Verification items for the finished model (mm, model axes). Face numbers are marked on the shaded views. A direction names the side the tool comes from. Round coordinates to 2 decimals unless told otherwise and drop trailing zeros. Order: outer loops, then holes, each group sorted by start corner. A loop starts at its lowest first (then second) coordinate and runs counter-clockwise, first axis right, second up. Notation, with made-up numbers: (75, 22.25) -> (108, 22.25) arc R35 cw to (108, 56.25) -> close; hole circle Ø4 at (-28, 4). An arc over 180 degrees is marked (long way). Return JSON: item names as keys, results as strings. Group by question number.
Item 1: Sectioned sample at D-D on z = 2.25. Record the cut outline in (x, y).
Item 2: Scan lines: probe 1 along Y at (x, z) = (0, 6.25); probe 2 along Y at (x, z) = (0, 3); probe 3 along X at (y, z) = (0, 3.75). Record each from-to range of solid material in increasing order. Write a range as from..to.
Item 3: Sectioned sample at B-B on x = -8. Record the cut outline in (y, z), plus the area to 4 significant figures.
Item 4: Depth check by flat-ended pin: pin 1 Ø1.5 at (x, z) = (7.5, -3) entering from +Y; pin 2 Ø1 at (y, z) = (-1, -1) entering from -X; pin 3 Ø3 at (x, z) = (-6, -4.5) entering from -Y. Enter the tip coordinate at first touch or a pass-through.
Item 5: Sectioned sample at A-A on z = 9. Record the cut outline in (x, y), plus the area to 3 significant figures.
Item 6: Access from +Z, -Z, +X, -X, +Y, -Y to the whole of each face (thin tool, end or side, straight path). Record for the marked faces 1, 2 and 3.
Item 7: Sectioned sample at C-C on y = 0. Record the cut outline in (x, z), plus the area to 3 significant figures.
Item 8: Draft check along X on the marked faces 4, 5, 6 and 7. Enter one of: pulls with the +X half, pulls with the -X half, needs draft (parallel to the pull), parting line crosses it, or undercut.
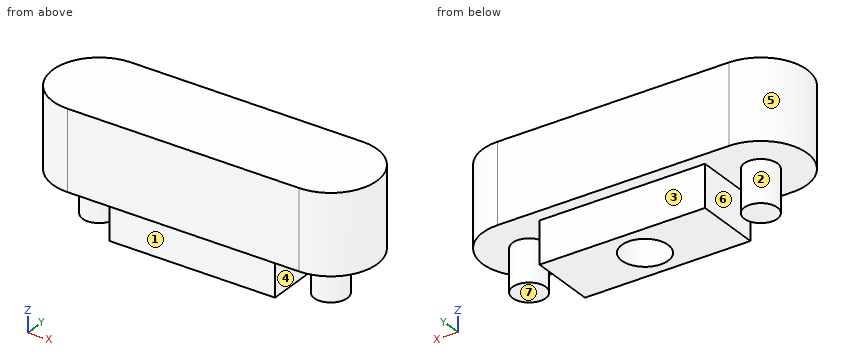
Autodesk Inventor part; units mm, degrees
ref_plane "YZ Plane" through (0, 0, 0) normal (1, 0, 0) x (0, 1, 0)
ref_plane "XZ Plane" through (0, 0, 0) normal (0, 1, 0) x (-1, 0, 0)
ref_plane "XY Plane" through (0, 0, 0) normal (0, 0, 1) x (1, 0, 0)
sketch "Sketch1" plane through (0, 0, 0) normal (0, 0, 1) x (1, 0, 0)
  circle A0 centre (17.5, 0) radius 2.5
  circle A1 centre (-17.5, 0) radius 2.5
  line L0 (17.5, -7) -> (-17.5, -7)
  arc A2 (-17.5, 7) -> (-17.5, -7) centre (-17.5, 0) ccw
  line L1 (-17.5, 7) -> (17.5, 7)
  arc A3 (17.5, -7) -> (17.5, 7) centre (17.5, 0) ccw
  line L2 (-12.5, -5) -> (12.5, -5)
  line L3 (12.5, 5) -> (-12.5, 5)
  circle A4 centre (0, 0) radius 3.5
  dimension "d0" = 2
  dimension "d1" = 17.5
  dimension "d2" = 7
extrude "Extrusion1" add sketch "Sketch1" along normal blind 10 contours A0 | A1 | L0 A2 L1 A3
sketch "Sketch2" plane through (0, 0, 10) normal (0, 0, 1) x (1, 0, 0)
  arc A0 (17.5, -7) -> (17.5, 7) centre (17.5, 0) ccw
  line L0 (-17.5, -7) -> (17.5, -7)
  arc A1 (-17.5, 7) -> (-17.5, -7) centre (-17.5, 0) ccw
  line L1 (17.5, 7) -> (-17.5, 7)
  point P0 (0, 0)
extrude "Extrusion2" add sketch "Sketch2" along normal blind 2
sketch "Sketch3" plane through (0, 0, 10) normal (0, 0, -1) x (-1, 0, 0)
  circle A0 centre (0, 0) radius 1.7
  dimension "d7" = 3.4
extrude "Extrusion3" add sketch "Sketch3" along normal blind 5
sketch "Sketch4" plane through (0, 0, 0) normal (0, 0, -1) x (-1, 0, 0)
  circle A0 centre (17.5, 0) radius 2.5
  line L0 (12.5, 5) -> (12.5, -5)
  line L1 (-12.5, 5) -> (12.5, 5)
  line L2 (12.5, -5) -> (-12.5, -5)
  line L3 (-12.5, -5) -> (-12.5, 5)
  circle A1 centre (0, 0) radius 3.5
  circle A2 centre (-17.5, 0) radius 2.5
extrude "Extrusion4" add sketch "Sketch4" along normal blind 6.35
properties part number "SpringHolderV1"
Recorded:
{
 "1": {"outline": "(-17.5, -7) -> (17.5, -7) arc R7 ccw to (17.5, 7) -> (-17.5, 7) arc R7 ccw to start; hole circle Ø7 at (0, 0)"},
 "2": {"probe 1": "-7..-3.5, -1.7..1.7, 3.5..7", "probe 2": "-7..-3.5, 3.5..7", "probe 3": "-24.5..-3.5, 3.5..24.5"},
 "3": {"outline": "(-7, 0) -> (-5, 0) -> (-5, -6.35) -> (5, -6.35) -> (5, 0) -> (7, 0) -> (7, 12) -> (-7, 12) -> close", "area": "231.5 mm²"},
 "4": {"pin 1": "y = 5", "pin 2": "x = -19.95", "pin 3": "y = -5"},
 "5": {"outline": "(-17.5, -7) -> (17.5, -7) arc R7 ccw to (17.5, 7) -> (-17.5, 7) arc R7 ccw to start; circle Ø3.4 at (0, 0); hole circle Ø7 at (0, 0)", "area": "615 mm²"},
 "6": {"face 1": "-Z, +X, -X, -Y", "face 2": "-Z", "face 3": "-Z, +X, -X, +Y"},
 "7": {"outline": "(-24.5, 0) -> (-20, 0) -> (-20, -6.35) -> (-15, -6.35) -> (-15, 0) -> (-12.5, 0) -> (-12.5, -6.35) -> (-3.5, -6.35) -> (-3.5, 10) -> (-1.7, 10) -> (-1.7, 5) -> (1.7, 5) -> (1.7, 10) -> (3.5, 10) -> (3.5, -6.35) -> (12.5, -6.35) -> (12.5, 0) -> (15, 0) -> (15, -6.35) -> (20, -6.35) -> (20, 0) -> (24.5, 0) -> (24.5, 12) -> (-24.5, 12) -> close", "area": "713 mm²"},
 "8": {"face 4": "undercut", "face 5": "pulls with the -X half", "face 6": "undercut", "face 7": "needs draft"}
}
